from build123d import *

# Parameters (mm, degrees)
BOSS_EXTRUDE1_DEPTH = 9
FILLET1_R           = 6
FILLET2_R           = 6
FILLET3_R           = 6
SKETCH4_R           = 1.5
CUT_EXTRUDE2_DEPTH  = 99.948249762


with BuildPart() as part:
    # Sketch1 → Boss-Extrude1 (new, symmetric)
    with BuildSketch(Plane(origin=(0, 0, 0), x_dir=(1, 0, 0), z_dir=(0, 1, 0))):
        Polygon((26.298098503, -33.68255382), (0, 0), (23.549059428, -4.630529132), (34.208885562, -27.565410034), (38.800851719, -33.702486103), (41.023010007, -30.384019108), (48.078540091, -41.414607796), (46.07366082, -44.408600496), (46.07366082, -84.588475064), (35.07366082, -84.588475064), (35.07366082, -77.588475064), (20.351319641, -51.449372742), (22.771974432, -47.270927217), (22.771974432, -37.270927217), align=None)
    extrude(amount=BOSS_EXTRUDE1_DEPTH, both=True)

    # Fillet1
    fillet1_edges = [part.edges().sort_by_distance(p)[0] for p in [
        (0, 0, 0),
        (23.549059428, 0, 4.630529132),
    ]]
    fillet(fillet1_edges, radius=FILLET1_R)

    # Fillet2
    fillet2_edges = [part.edges().sort_by_distance(p)[0] for p in [
        (22.771974432, 0, 47.270927217),
        (22.771974432, 0, 37.270927217),
    ]]
    fillet(fillet2_edges, radius=FILLET2_R)

    # Fillet3
    fillet3_edges = [part.edges().sort_by_distance(p)[0] for p in [
        (35.07366082, 0, 84.588475064),
    ]]
    fillet(fillet3_edges, radius=FILLET3_R)

    # Sketch4 → Cut-Extrude2 (cut, through all)
    with BuildSketch(Plane(origin=(0, 9, 0), x_dir=(1, 0, 0), z_dir=(0, 1, 0))):
        with Locations(Location((14.632977879, -8.992224551, 0), (0, 0, 270))):
            Circle(SKETCH4_R)
    extrude(amount=-CUT_EXTRUDE2_DEPTH, mode=Mode.SUBTRACT)


solid = part.part
Could you check a few things on this model? Use its own coordinates, in mm. A direction names the side the tool comes from. Coordinates: 2 decimals unless noted, no trailing zeros. Write each loop counter-clockwise with the first axis right and the second up, starting at its lowest first coordinate (ties: lowest second). Pieces come first, ordered by that corner, then holes. Notation, with made-up numbers: M -7,88 L 6,88 A17 cw 6,113 Z; hole C -29.5,10.5 d7. An arc over 180 degrees is marked long. One line per question, with ' | ' between items.
1) If we mould it in two halves opening along Z, with no side actions, what happens to faces 1 (the face through (9.468, -0.126, 5.938)), 2 (the face through (46.074, 0, 64)), 3 (the face through (16.12, 0.13, 8.8)), 4 (the face through (29.457, 0.126, 17.341))? For each: released by +Z, released by -Z, zero draft, split by the parting line, or undercut.
Checks:
face 1: split by the parting line | face 2: zero draft | face 3: undercut | face 4: released by -Z
2) Imagine slicing it at C-C, the plane z = 42.5. Write out the boundary of the cut face in (x, y), and give its area (3 significant figures).
Checks:
outline: M 22.77,-9 L 47.35,-9 L 47.35,9 L 22.77,9 Z | area: 442 mm²
3) Imagine slicing it at A-A, the plane y = -1. Write out the boundary of the cut face in (x, z).
Checks:
outline: M 9.9,12.68 A6 ccw 15.79,3.1 L 20.55,4.04 A6 ccw 24.84,7.4 L 34.21,27.57 L 38.8,33.7 L 41.02,30.38 L 48.08,41.41 L 46.07,44.41 L 46.07,84.59 L 41.07,84.59 A6 ccw 35.07,78.59 L 35.07,77.59 L 20.35,51.45 L 21.96,48.67 A6 cw 22.77,45.66 L 22.77,39.73 A6 ccw 24.49,35.52 L 26.3,33.68 Z; hole C 14.63,8.99 d3
4) I need wall thicknesses on probe 1 along X at (y, z) = (-2.25, 45.5); probe 2 along Z at (x, y) = (23.5, -1); probe 3 along Z at (x, y) = (20.5, 3.25). Which ranges of each line are inside material? Lowest first, please. Write a range as [from, to].
Checks:
probe 1: [22.77, 46.07] | probe 2: [5.55, 30.1], [36.86, 57.04] | probe 3: [4.03, 26.26], [51.19, 51.71]
5) Imagine slicing it at B-B, the plane x = 42. Write out the boundary of the cut face in (y, z).
Checks:
outline: M -9,31.91 L 9,31.91 L 9,84.59 L -9,84.59 Z
6) For pin 1 Ø3 at (x, y) = (28.5, -3) entering from +Z; pin 2 Ø10 at (y, z) = (-6, 17) entering from +X; pin 3 Ø1.5 at (x, y) = (15, 0.5) entering from -Z; pin 4 Ø3 at (y, z) = (2.5, 42.5) entering from -X, each with a flat end and sliding along its axis, tell me the tip position at first contact or that it passes through.
Checks:
pin 1: z = 68.58 | pin 2: x = 31.62 | pin 3: z = 2.99 | pin 4: x = 22.77
7) For faces 5 (the face through (33, 9, 43)), 6 (the face through (23.231, 0.126, 37.424)), 7 (the face through (36.47, 0.13, 30.59)), which set-ups out of +Z, -Z, +X, -X, +Y, -Y let a thin tool reach every point of the face, with its end or its side?
Checks:
face 5: +Z, -Z, +X, -X, +Y | face 6: -X, +Y, -Y | face 7: -Z, +Y, -Y
